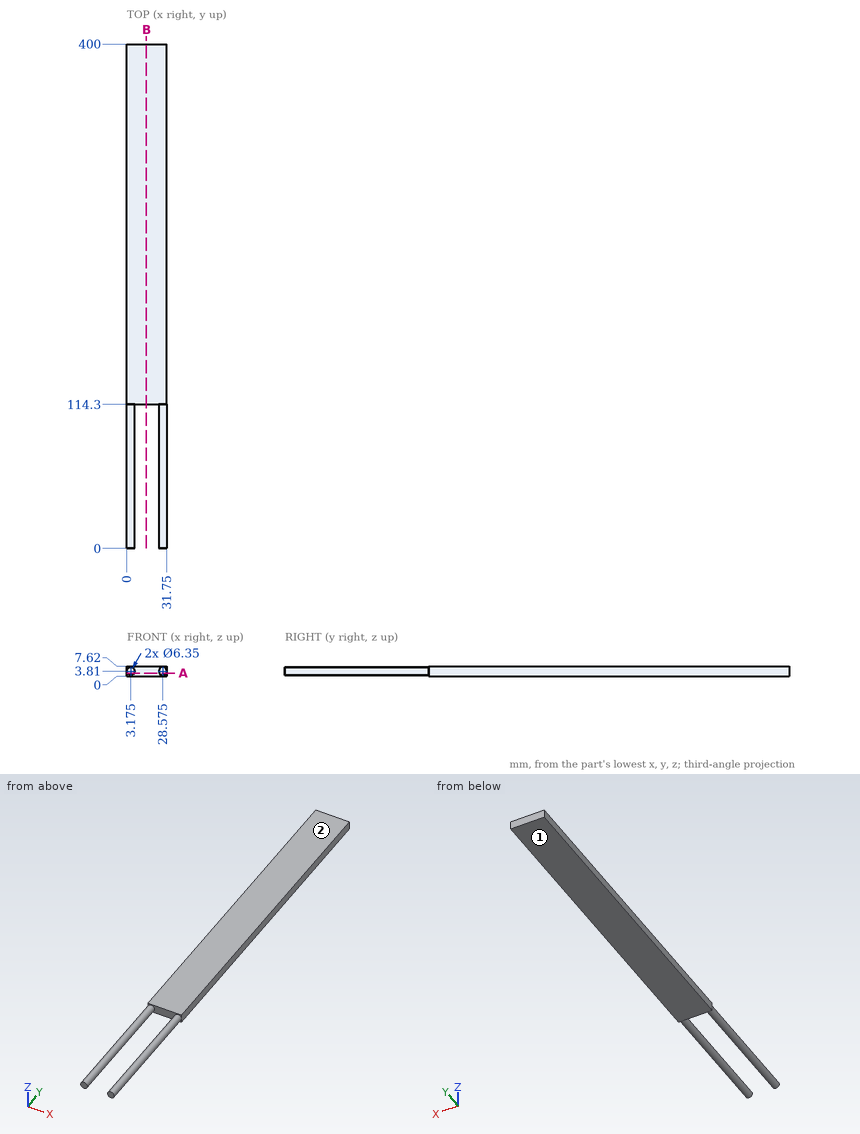
Print and shaded views of the part. All mm, measured from the part's lowest x, y and z. Coordinates: 2 decimals unless noted, no trailing zeros. Order: outer loops, then holes, each group sorted by start corner. A loop starts at its lowest first (then second) coordinate and runs counter-clockwise, first axis right, second up. Notation, with made-up numbers: (-3.5, -4.75) - (53.5, -4.75) arc R30 cw to (53.5, 20.25) - close; hole circle Ø3 at (6.25, -4). An arc over 180 degrees is marked (long way). Return JSON: item names as keys, results as strings. Group by question number.
Item 1: Drill centre lines: probe 1 along X at (y, z) = (24.5, 4.25); probe 2 along Y at (x, z) = (17, 7.25); probe 3 along X at (y, z) = (41, 5). Where is each one in solid material? Low to high. Write a range as from..to.
Item 2: Cut at A-A (z = 2.25). List the corners of the cut face in (x, y), plus the area to 3 significant figures.
Item 3: Pin check, flat tips, straight feed: pin 1 (12 mm diameter, centred on x = 12.5, y = 66.5, fed in from +Z); pin 2 (4 mm diameter, centred on x = 10, z = 4.5, fed in from -Y); pin 3 (12 mm diameter, centred on x = 26, y = 71, fed in from -Z) (3 decimals); pin 4 (4 mm diameter, centred on x = 6, y = 225.5, fed in from -Z). Stop position of each tip, or through.
Item 4: Cut at B-B (x = 15.5). List the corners of the cut face in (y, z).
Item 5: Pull direction Z, two halves, no side cores. Call the marked faces 1 and 2: pulls with the +Z half, pulls with the -Z half, needs draft (parallel to the pull), parting line crosses it, or undercut.
Check values:
{
 "1": {"probe 1": "x = 0.03..6.32, 25.43..31.72", "probe 2": "y = 114.3..400", "probe 3": "x = 0.23..6.12, 25.63..31.52"},
 "2": {"outline": "(0, 114.3) - (0.41, 114.3) - (0.41, 0) - (5.94, 0) - (5.94, 114.3) - (25.81, 114.3) - (25.81, 0) - (31.34, 0) - (31.34, 114.3) - (31.75, 114.3) - (31.75, 400) - (0, 400) - close", "area": "10,300 mm2"},
 "3": {"pin 1": "passes through", "pin 2": "stops at y = 114.3", "pin 3": "stops at z = 0.635", "pin 4": "stops at z = 0"},
 "4": {"outline": "(114.3, 0) - (400, 0) - (400, 7.62) - (114.3, 7.62) - close"},
 "5": {"face 1": "pulls with the -Z half", "face 2": "pulls with the +Z half"}
}
